```python
from build123d import *

# Parameters (mm, degrees)
CROQUIS2_W                   = 160
CROQUIS2_H                   = 160
CROQUIS2_W_2                 = 140
CROQUIS2_H_2                 = 140
SALIENTE_EXTRUIR1_DEPTH      = 10
CROQUIS4_W                   = 10
CROQUIS4_H                   = 10
SALIENTE_EXTRUIR2_DEPTH      = 140
SALIENTE_EXTRUIR2_DEPTH_BACK = 10
CROQUIS7_W                   = 160
CROQUIS7_H                   = 160
CROQUIS7_W_2                 = 140
CROQUIS7_H_2                 = 140
SALIENTE_EXTRUIR3_DEPTH      = 10
CROQUIS8_W                   = 63
CROQUIS8_H                   = 12
CROQUIS8_R                   = 2.5
SALIENTE_EXTRUIR4_DEPTH      = 5
CROQUIS9_W                   = 174.167702824
CROQUIS9_H                   = 180.53552259
CORTAR_EXTRUIR2_DEPTH        = 161
CROQUIS10_R                  = 2.5
CORTAR_EXTRUIR3_DEPTH        = 4


with BuildPart() as part:
    # Croquis2 → Saliente-Extruir1 (new body)
    with BuildSketch(Plane.XY):
        with Locations((80, -80)):
            Rectangle(CROQUIS2_W, CROQUIS2_H)
        with Locations((80, -80)):
            Rectangle(CROQUIS2_W_2, CROQUIS2_H_2, mode=Mode.SUBTRACT)
    extrude(amount=SALIENTE_EXTRUIR1_DEPTH)

    # Croquis4 → Saliente-Extruir2 (add, two sides)
    with BuildSketch(Plane.XY.offset(10)) as saliente_extruir2_sk:
        with Locations((5, -5)):
            Rectangle(CROQUIS4_W, CROQUIS4_H)
        with Locations((155, -5)):
            Rectangle(CROQUIS4_W, CROQUIS4_H)
        with Locations((155, -155)):
            Rectangle(CROQUIS4_W, CROQUIS4_H)
        with Locations((5, -155)):
            Rectangle(CROQUIS4_W, CROQUIS4_H)
    extrude(amount=SALIENTE_EXTRUIR2_DEPTH)
    extrude(saliente_extruir2_sk.sketch, amount=-SALIENTE_EXTRUIR2_DEPTH_BACK)

    # Croquis7 → Saliente-Extruir3 (add)
    with BuildSketch(Plane.XY.offset(150)):
        with Locations((80, -80)):
            Rectangle(CROQUIS7_W, CROQUIS7_H)
        with Locations((80, -80)):
            Rectangle(CROQUIS7_W_2, CROQUIS7_H_2, mode=Mode.SUBTRACT)
    extrude(amount=SALIENTE_EXTRUIR3_DEPTH)

    # Croquis8 → Saliente-Extruir4 (add)
    with BuildSketch(Plane.XY.offset(160)):
        with Locations((31.5, -80)):
            Rectangle(CROQUIS8_W, CROQUIS8_H)
        with Locations((55, -80)):
            Circle(CROQUIS8_R, mode=Mode.SUBTRACT)
        with Locations((128.5, -80)):
            Rectangle(CROQUIS8_W, CROQUIS8_H)
        with Locations((105, -80)):
            Circle(CROQUIS8_R, mode=Mode.SUBTRACT)
    extrude(amount=-SALIENTE_EXTRUIR4_DEPTH)

    # Croquis9 → Cortar-Extruir2 (cut, through all)
    with BuildSketch(Plane.ZY):
        with Locations((97.083851412, -84.953806067)):
            Rectangle(CROQUIS9_W, CROQUIS9_H)
    extrude(amount=-CORTAR_EXTRUIR2_DEPTH, mode=Mode.SUBTRACT)

    # Croquis10 → Cortar-Extruir3 (cut)
    with BuildSketch(Plane.XY.offset(10)):
        with Locations((5, -155)):
            Circle(CROQUIS10_R)
        with Locations((5, -5)):
            Circle(CROQUIS10_R)
        with Locations((155, -5)):
            Circle(CROQUIS10_R)
        with Locations((155, -155)):
            Circle(CROQUIS10_R)
    extrude(amount=-CORTAR_EXTRUIR3_DEPTH, mode=Mode.SUBTRACT)


solid = part.part
```
Could you check a few things on this model? Use its own coordinates, in mm. A direction names the side the tool comes from. Coordinates: 2 decimals unless noted, no trailing zeros. Write each loop counter-clockwise with the first axis right and the second up, starting at its lowest first coordinate (ties: lowest second). Pieces come first, ordered by that corner, then holes. Notation, with made-up numbers: (-12, 84) -> (-1, 84) arc R28 cw to (-1, 102) -> close; hole circle Ø11 at (6, 89.25). An arc over 180 degrees is marked (long way). Return JSON: item names as keys, results as strings.
(1) I need wall thicknesses on L1, parallel to Y at x = 5, z = 8.1; L2, parallel to X at y = -155, z = 8.7; L3, parallel to X at y = -127.5, z = 7.75. Which ranges of each line are inside material? Lowest first, please.
Numbers:
{"L1": "y = -160 to -157.5, -152.5 to -7.5, -2.5 to 0", "L2": "x = 0 to 2.5, 7.5 to 152.5, 157.5 to 160", "L3": "x = 0 to 10, 150 to 160"}
(2) Imagine slicing it at B-B, the plane z = 8. Please give me the cut outline in (x, y), then the cut area to 3 significant figures.
Numbers:
{"outline": "(0, -160) -> (160, -160) -> (160, 0) -> (0, 0) -> close; hole circle Ø5 at (5, -155); hole circle Ø5 at (5, -5); hole (10, -150) -> (150, -150) -> (150, -10) -> (10, -10) -> close; hole circle Ø5 at (155, -155); hole circle Ø5 at (155, -5)", "area": "5,920 mm2"}
(3) Imagine slicing it at C-C, the plane y = -117. Please give me the cut outline in (x, z).
Numbers:
{"outline": "(0, 0) -> (10, 0) -> (10, 10) -> (0, 10) -> close; (150, 0) -> (160, 0) -> (160, 10) -> (150, 10) -> close"}
(4) I'm going to push a flat-ended pin straight in: pin 1 (2.5 mm diameter, centred on x = 154, y = -154.5, fed in from +Z). Where does the tip first touch, or does it pass through?
Numbers:
{"pin 1": "stops at z = 6"}
(5) Imagine slicing it at A-A, the plane x = 147. Please give me the cut outline in (y, z), then the cut area to 3 significant figures.
Numbers:
{"outline": "(-160, 0) -> (-150, 0) -> (-150, 10) -> (-160, 10) -> close; (-10, 0) -> (0, 0) -> (0, 10) -> (-10, 10) -> close", "area": "200 mm2"}
(6) Imagine slicing it at D-D, the plane x = 5. Please give me the cut outline in (y, z), then the cut area to 3 significant figures.
Numbers:
{"outline": "(-160, 0) -> (0, 0) -> (0, 10) -> (-2.5, 10) -> (-2.5, 6) -> (-7.5, 6) -> (-7.5, 10) -> (-152.5, 10) -> (-152.5, 6) -> (-157.5, 6) -> (-157.5, 10) -> (-160, 10) -> close", "area": "1,560 mm2"}
(7) We'd pull the mould along Y, two halves only. Please class faces 4 (the flat face through (79, -10, 5)), 5 (the flat face through (9, -80, 0)), 6 (the flat face through (79, 0, 5)), 7 (the flat face through (79, -160, 5)): +Y half, -Y half, draft (parallel to the pull), parting line (faces both ways), or undercut.
Numbers:
{"face 4": "undercut", "face 5": "draft", "face 6": "+Y half", "face 7": "-Y half"}
(8) Which directions (+Z, -Z, +X, -X, +Y, -Y) give clear straight access to the entire face, cutting with the end or side of a thin tool? Please do faces 1 (the flat face through (160, -81, 5)), 2 (the cylindrical face through (157.385, -4.249, 8.028)), 3 (the flat face through (79, -150, 5)).
Numbers:
{"face 1": "+Z, -Z, +X, +Y, -Y", "face 2": "+Z", "face 3": "+Z, -Z"}
